Autodesk Inventor part; units mm, degrees
ref_plane "YZ Plane" through (0, 0, 0) normal (1, 0, 0) x (0, 1, 0)
ref_plane "XZ Plane" through (0, 0, 0) normal (0, 1, 0) x (-1, 0, 0)
ref_plane "XY Plane" through (0, 0, 0) normal (0, 0, 1) x (1, 0, 0)
sketch "Sketch1" plane through (0, 0, 0) normal (0, 0, 1) x (1, 0, 0)
  line L0 (0, 0) -> (35, 0)
  line L1 (35, 0) -> (35, -5)
  line L2 (35, -5) -> (0, -5)
  line L3 (0, -5) -> (0, 0)
  dimension "d0" = 35
  dimension "d1" = 5
extrude "Extrusion1" add sketch "Sketch1" along normal blind 18
sketch "Sketch2" plane through (0, 0, 18) normal (0, 0, 1) x (1, 0, 0)
  line L0 (0, 0) -> (0, -5)
  line L1 (0, 0) -> (35, 0)
  point P0 (2.5, -2.5)
  dimension "d4" = 2.5
  dimension "d5" = 2.5
hole "Hole1" at (2.5, -2.5, 18) direction (0, 0, -1) diameter 3.1 end through all
fillet "Fillet1" radius 1 2 edges at (35, -5, 9) (35, 0, 9)
fillet "Fillet2" radius 2.5 2 edges at (0, -5, 9) (0, 0, 9)
sketch "Sketch3" plane through (0, 0, 18) normal (0, 0, 1) x (1, 0, 0)
  circle A0 centre (2.5, -2.5) radius 1.55 construction
  line L0 (2.5, -5) -> (34, -5) construction
  line L1 (34, 0) -> (2.5, 0) construction
  line L2 (35, -4) -> (35, -1) construction
  point P0 (0, 0)
  point P1 (32.5, -2.5)
  dimension "d15" = 2.5
  dimension "d16" = 2.5
  dimension "d17" = 5
hole "Hole2" at (32.5, -2.5, 18) direction (0, 0, -1) diameter 2 depth 11 tip angle 118
properties part number "porte"
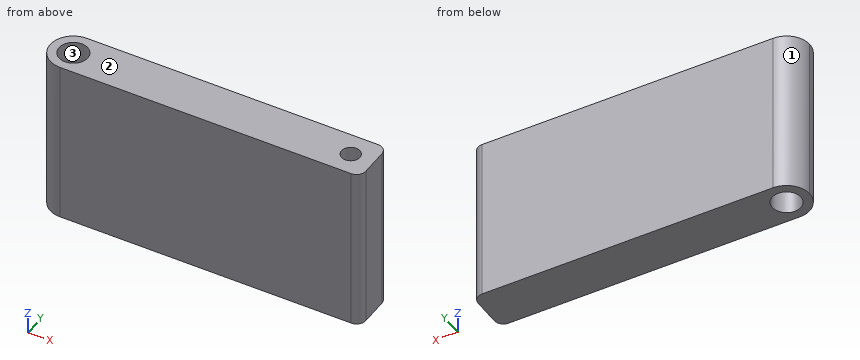
The listing builds one solid part. Answer for the finished solid, in the listing's coordinates (mm). Face numbers are marked on the shaded views. Coordinates: 2 decimals unless noted, no trailing zeros. Loops run counter-clockwise (first coordinate to the right, second up) from the corner with the lowest first, then second, coordinate; pieces in that order, holes last. Notation, with made-up numbers: M -18.75,66.5 L 39.25,66.5 A18 ccw 39.25,97.5 Z; hole C 71.25,1 d2. An arc over 180 degrees is marked long. Answer as CSV lines item,"result". Start each with the question number.
(1) The mould has two halves that part along Y. Classify the marked faces 1, 2 and 3: pulls with the +Y half, pulls with the -Y half, needs draft (parallel to the pull), parting line crosses it, or undercut.
(2) The part is cut by section C-C (y = -0.45). Give the vertices of the cut face in (x, z).
(3) Find the intervals of material crossed by L1, parallel to X at y = -2.5, z = 15; L2, parallel to Y at x = 32.5, z = 14.5; L3, parallel to X at y = -2.55, z = 4.25, in increasing order. Write a range as [from, to].
(4) The part is cut by section B-B (y = -4.6). Give the vertices of the cut face in (x, z).
(5) Given pin 1 (2.5 mm diameter, centred on x = 32.5, y = -2.5, fed in from +Z), flat-ended and moving along its own axis, determine where the tip first touches the part or whether it passes through.
(6) The part is cut by section A-A (z = 8.75). State how many separate pieces and enclosed holes the cut face has, and give its area (3 significant figures).
Determined:
1,face 1,"pulls with the +Y half"
1,face 2,"needs draft"
1,face 3,"undercut"
2,outline,"M 1.07,0 L 34.84,0 L 34.84,18 L 1.07,18 Z"
3,L1,"[0, 0.95], [4.05, 31.5], [33.5, 35]"
3,L2,"[-5, -3.5], [-1.5, 0]"
3,L3,"[0, 0.95], [4.05, 35]"
4,outline,"M 1.14,0 L 34.8,0 L 34.8,18 L 1.14,18 Z"
5,pin 1,"z = 18"
6,separate pieces,"1"
6,enclosed holes,"2"
6,area,"161 mm2"
